```python
from build123d import *

# Parameters (mm, degrees)
F2_T        = -1.27
F3_SIZE     = 0.254
F4_R        = 6.9696549561
F4_R_2      = 6.3199888533
F5_DEPTH    = 0.254
F7_S5_R     = 11.5270866081
F7_T6_DEPTH = 20


# Not quite as in the source:
# - a fillet or chamfer that OpenCascade refuses, or shapes differently, is made with other operations: its cross-section is extruded or revolved along the edge and cut away or added


with BuildPart() as f1:
    # F0 (on Front) → F1 (revolve)
    with BuildSketch(Plane.XZ):
        Polygon((0, 56.7248165607), (0, 0), (12.7805937082, 0), (12.7805937082, 1.5856500249), (11.5270866081, 1.5856500249), (11.5270866081, 2.6958733797), (12.7805937082, 2.6958733797), (12.7805937082, 56.7248165607), align=None)
    revolve(axis=Axis((0, 0, 24.1605676711), (0, 0, -1)))

    # F2
    f2_openings = [f1.faces().sort_by_distance(p)[0] for p in [
        (0, 0, 56.724817),
    ]]
    offset(amount=F2_T, openings=f2_openings, kind=Kind.INTERSECTION)

    # F3
    f3_edges = [f1.edges().sort_by_distance(p)[0] for p in [
        (-12.780594, 0, 0),
    ]]
    chamfer(f3_edges, length=F3_SIZE)

    # F4 (on face) → F5 (cut)
    with BuildSketch(Plane(origin=(0, 0, 0), x_dir=(1, 0, 0), z_dir=(0, 0, -1))):
        Circle(F4_R)
        Circle(F4_R_2, mode=Mode.SUBTRACT)
    extrude(amount=-F5_DEPTH, mode=Mode.SUBTRACT)

    # F6: fillet of radius 0.762 on 2 edges, made by hand

    # F6_s1 → F6_t2 (revolve, cut)
    with BuildSketch(Plane.XZ):
        with BuildLine():
            ThreePointArc((6.3199888533, 0.254), (6.0631127843, 0.066392352), (5.752027587, 0))
            Line((5.752027587, 0), (6.3199888533, 0))
            Line((6.3199888533, 0), (6.3199888533, 0.254))
        make_face()
    revolve(axis=Axis((0, 0, 0), (0, 0, -1)), mode=Mode.SUBTRACT)

    # F6_s3 → F6_t4 (revolve, cut)
    with BuildSketch(Plane.XZ):
        with BuildLine():
            ThreePointArc((7.5376162224, 0), (7.226531025, 0.066392352), (6.9696549561, 0.254))
            Line((6.9696549561, 0.254), (6.9696549561, 0))
            Line((6.9696549561, 0), (7.5376162224, 0))
        make_face()
    revolve(axis=Axis((0, 0, 0), (0, 0, -1)), mode=Mode.SUBTRACT)

    # F7: chamfer of 2.54 on 1 edges, made by hand


with BuildPart() as f7_tool2:
    # F7_s3 → F7_t4 (revolve)
    with BuildSketch(Plane.XZ):
        Polygon((10.2405937082, 2.6958733797), (12.7805937082, 5.2358733797), (12.7805937082, 2.6958733797), align=None)
    revolve(axis=Axis((0, 0, 2.6958733797), (0, 0, -1)))

    # F7_s5 → F7_t6 (cut, symmetric)
    with BuildSketch(Plane.XY.offset(4)):
        Circle(F7_S5_R)
    extrude(amount=F7_T6_DEPTH, both=True, mode=Mode.SUBTRACT)


with BuildPart() as f1_1:
    add(f1.part)

    # F7_t1: cut F7_tool2
    add(f7_tool2.part, mode=Mode.SUBTRACT)


solid = f1_1.part
```
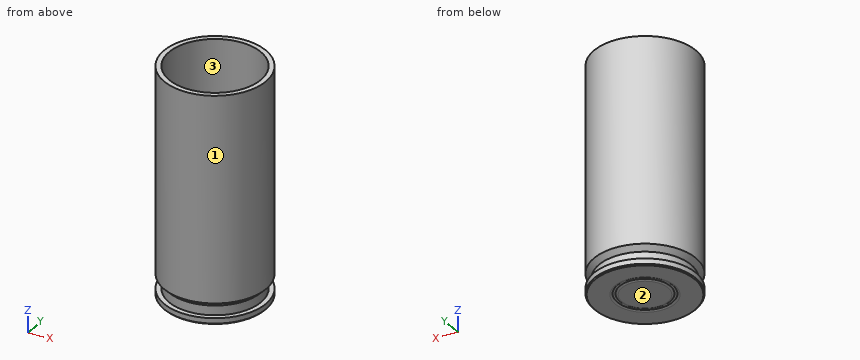
The listing builds one solid part. Answer for the finished solid, in the listing's coordinates (mm). Face numbers are marked on the shaded views. Coordinates: 2 decimals unless noted, no trailing zeros. Write each loop counter-clockwise with the first axis right and the second up, starting at its lowest first coordinate (ties: lowest second). Pieces come first, ordered by that corner, then holes. Notation, with made-up numbers: M 0.25,2.5 L 10.25,2.5 A29 cw 10.25,41.5 Z; hole C -24.75,67 d6. An arc over 180 degrees is marked long. Use a Markdown table: item, result. Add a question column.
1. For a pull along Y with two mould halves and no side action, classify the marked faces 1, 2 and 3 as +Y half, -Y half, draft (parallel to the pull), parting line (faces both ways), or undercut.
2. Given P1, Ø6, axis at x = 2.5, y = -4, coming from the +Z side; P2, Ø3, axis at y = 2.5, z = 21.5, coming from the +X side; P3, Ø8, axis at x = 1, y = 6.5, coming from the +Z side, each flat-ended and moving along its own axis, determine where each tip first touches the part or whether it passes through.
3. Straight lines are drawn through the part: line 1 along Y through (x, z) = (0, 2.7); line 2 along Y through (x, z) = (0, 29.5); line 3 along Z through (x, y) = (0.25, 0.75). For each, find the intervals that lie inside material, in ascending order. Write a range as [from, to].
4. Section C-C (z = 26.5) is taken. Give the vertices of the cut face in (x, y), plus the area to 3 significant figures.
Data:
| question | item | result |
|---|---|---|
| 1 | face 1 | parting line |
| 1 | face 2 | draft |
| 1 | face 3 | undercut |
| 2 | P1 | stops at z = 1.27 |
| 2 | P2 | stops at x = 12.74 |
| 2 | P3 | stops at z = 3.97 |
| 3 | line 1 | y = [-11.53, -10.26], [10.26, 11.53] |
| 3 | line 2 | y = [-12.78, -11.51], [11.51, 12.78] |
| 3 | line 3 | z = [0, 1.27] |
| 4 | outline | C 0,0 d25.56; hole C 0,0 d23.02 |
| 4 | area | 96.9 mm2 |
